from build123d import *

# Parameters (mm, degrees)
SKETCH4_R           = 34.2265
BOSS_EXTRUDE1_DEPTH = 63.5
SKETCH5_R           = 34.2265
BOSS_EXTRUDE2_DEPTH = 31.75
CUT_EXTRUDE1_REACH  = 36.227
SKETCH8_R           = 3.175


with BuildPart() as part:
    # Sketch1 → Revolve1 (revolve)
    with BuildSketch(Plane.XY):
        Polygon((-66.802, -34.2265), (-31.75, -34.2265), (-31.75, -30.0863), (-66.802, -30.3149), align=None)
        Polygon((66.802, -30.3149), (31.75, -30.0863), (31.75, -34.2265), (66.802, -34.2265), align=None)
    revolve(axis=Axis((-66.802, 0, 0), (1, 0, 0)))



with BuildPart() as body_2:
    # Sketch2 → Revolve2 (revolve)
    with BuildSketch(Plane.XY):
        Polygon((30.3149, 66.802), (30.0863, 31.75), (34.2265, 31.75), (34.2265, 66.802), align=None)
    revolve(axis=Axis((0, 0, 0), (0, 1, 0)))


with BuildPart() as part_1:
    add(part.part)

    add(body_2.part)  # Boss-Extrude1 merges body 2
    # Sketch4 → Boss-Extrude1 (add)
    with BuildSketch(Plane(origin=(-31.75, 0, 0), x_dir=(0, 0, -1), z_dir=(1, 0, 0))):
        Circle(SKETCH4_R)
    extrude(amount=BOSS_EXTRUDE1_DEPTH)

    # Sketch5 → Boss-Extrude2 (add)
    with BuildSketch(Plane.XZ.offset(-31.75)):
        Circle(SKETCH5_R)
    extrude(amount=BOSS_EXTRUDE2_DEPTH)

    # Sketch6 → Cut-Revolve1 (revolve, cut)
    with BuildSketch(Plane.XY):
        Polygon((-66.802, -30.3149), (-31.75, -30.0863), (-31.75, -26.2509), (31.75, -26.2509), (31.75, -30.0863), (66.802, -30.3149), (66.802, 0), (-66.802, 0), align=None)
    revolve(axis=Axis((66.802, 0, 0), (-1, 0, 0)), mode=Mode.SUBTRACT)

    # Sketch7 → Cut-Revolve2 (revolve, cut)
    with BuildSketch(Plane.XY):
        Polygon((30.3149, 66.802), (30.0863, 31.75), (26.2509, 31.75), (26.2509, 0), (0, 0), (0, 66.802), align=None)
    revolve(axis=Axis((0, 0, 0), (0, 1, 0)), mode=Mode.SUBTRACT)

    # Sketch8 → Cut-Extrude1 (cut, up to next)
    with BuildSketch(Plane(origin=(0, 0, 0), x_dir=(1, 0, 0), z_dir=(0, 1, 0)), mode=Mode.PRIVATE) as cut_extrude1_sk1:
        with Locations((35.71875, 0)):
            Circle(SKETCH8_R)
    cut_extrude1_tool1 = extrude(cut_extrude1_sk1.sketch, amount=-CUT_EXTRUDE1_REACH, mode=Mode.PRIVATE) & part_1.part
    add(cut_extrude1_tool1.solids().sort_by_distance((35.71875, 0, 0))[0], mode=Mode.SUBTRACT)
    # Sketch8 → Cut-Extrude1 (cut, up to next)
    with BuildSketch(Plane(origin=(0, 0, 0), x_dir=(1, 0, 0), z_dir=(0, 1, 0)), mode=Mode.PRIVATE) as cut_extrude1_sk2:
        with Locations((-35.71875, 0)):
            Circle(SKETCH8_R)
    cut_extrude1_tool2 = extrude(cut_extrude1_sk2.sketch, amount=-CUT_EXTRUDE1_REACH, mode=Mode.PRIVATE) & part_1.part
    add(cut_extrude1_tool2.solids().sort_by_distance((-35.71875, 0, 0))[0], mode=Mode.SUBTRACT)


solid = part_1.part
Geometry: final body of the model. Coordinates: model frame, mm. A direction names the side the tool comes from. Round coordinates to 2 decimals unless told otherwise and drop trailing zeros. Order: outer loops, then holes, each group sorted by start corner. A loop starts at its lowest first (then second) coordinate and runs counter-clockwise, first axis right, second up. Notation, with made-up numbers: (0, -40) - (4, -40) arc R18 ccw to (4, -28) - close; hole circle Ø8 at (49.25, 18). An arc over 180 degrees is marked (long way). Write each question's results on one line, items separated by ' | '.
Item 1: First-contact query: pin 1 Ø3.5 at (y, z) = (25.5, -3.5) entering from -X; pin 2 Ø5 at (x, z) = (1.5, -25) entering from +Y; pin 3 Ø3.5 at (y, z) = (27.5, 3.5) entering from +X. Flat tips, straight axial feed; report the tip coordinate or a pass-through.
Completed:
pin 1: x = -31.75 | pin 2: y = 31.75 | pin 3: x = 31.75
Item 2: Section C-C, the plane x = -54.5. Return the cut outline in (y, z).
Completed:
outline: circle Ø68.45 at (0, 0); hole circle Ø60.47 at (0, 0)
Item 3: Reachability of faces 1 (the cylindrical face through (-32.69, -32.06, -0.95)), 2 (the flat face through (66.802, 20, 23)), 3 (the cylindrical face through (14.112, 22.708, -22.135)) from +Z, -Z, +X, -X, +Y, -Y: full face, straight path, thin tool, end or side. Return the list, or none.
Completed:
face 1: -Y | face 2: +Z, -Z, +X, +Y, -Y | face 3: +Y
Item 4: Section A-A, the plane z = -15. State how many separate pieces and enclosed holes the cut face has, and give its area (3 significant figures).
Completed:
separate pieces: 3 | enclosed holes: 0 | area: 1,750 mm^2
Item 5: Section B-B, the plane x = 58.5. Return the cut outline in (y, z), and give its area (3 significant figures).
Completed:
outline: circle Ø68.45 at (0, 0); hole circle Ø60.52 at (0, 0) | area: 803 mm^2
Item 6: Mould query, pull axis Z, two halves, no side actions, for faces 4 (the cylindrical face through (32.646, 41.291, 10.281)), 5 (the flat face through (-66.802, -20, 23)), 6 (the cylindrical face through (38.75, -32.06, -0.95)). Classes: pulls with the +Z half, pulls with the -Z half, needs draft (parallel to the pull), parting line crosses it, or undercut.
Completed:
face 4: parting line crosses it | face 5: needs draft | face 6: undercut
Item 7: Material intervals for line 1 along Z through (x, y) = (0.5, 26); line 2 along Y through (x, z) = (41, 1.5); line 3 along Y through (x, z) = (6.5, 0), sorted ascending. Write a range as [from, to].
Completed:
line 1: [-34.22, -26.25], [26.25, 34.22] | line 2: [-34.19, -30.11], [30.11, 34.19] | line 3: [-34.23, -26.25]
